```python
from build123d import *

# Parameters (mm, degrees)
SKETCH1_R           = 7.875
BOSS_EXTRUDE1_DEPTH = 1
SKETCH2_R           = 0.85
CUT_EXTRUDE1_DEPTH  = 12.181737343
SKETCH3_R           = 0.65
CUT_EXTRUDE2_DEPTH  = 11


with BuildPart() as part:
    # Sketch1 → Boss-Extrude1 (new body)
    with BuildSketch(Plane(origin=(0, 0, 0), x_dir=(1, 0, 0), z_dir=(0, 1, 0))):
        with Locations(Location((0, 0, 0), (0, 0, 270))):
            Circle(SKETCH1_R)
    extrude(amount=BOSS_EXTRUDE1_DEPTH)

    # Sketch2 → Cut-Extrude1 (cut, through all)
    with BuildSketch(Plane(origin=(0, 1, 0), x_dir=(1, 0, 0), z_dir=(0, 1, 0))):
        with Locations(Location((0, 6.125, 0), (0, 0, 270))):
            Circle(SKETCH2_R)
        with Locations(Location((0, -6.125, 0), (0, 0, 90))):
            Circle(SKETCH2_R)
    extrude(amount=-CUT_EXTRUDE1_DEPTH, mode=Mode.SUBTRACT)

    # Sketch3 → Cut-Extrude2 (cut)
    with BuildSketch(Plane(origin=(0, 1, 0), x_dir=(1, 0, 0), z_dir=(0, 1, 0))):
        with Locations(Location((0.503115295, 1.65, 0), (0, 0, 270))):
            Circle(SKETCH3_R)
        with Locations(Location((0.503115295, -1.65, 0), (0, 0, 270))):
            Circle(SKETCH3_R)
    extrude(amount=-CUT_EXTRUDE2_DEPTH, mode=Mode.SUBTRACT)


solid = part.part
```
Part model, mm, in its own coordinate system. Round coordinates to 2 decimals unless told otherwise and drop trailing zeros. Order: outer loops, then holes, each group sorted by start corner. A loop starts at its lowest first (then second) coordinate and runs counter-clockwise, first axis right, second up. Notation, with made-up numbers: M 42.5,-11 L 91.5,-11 A14 cw 91.5,-6 Z; hole C 5,78 d7. An arc over 180 degrees is marked long. Answer in a Markdown table with one row per item. Add a question column.
Q1. Cut at B-B on y = 0.75. Give the cut face in (x, z) (3 decimals).
Q2. Cut at A-A on z = -5.5. Give the cut face in (x, y), and give its area (3 significant figures).
Q3. Cut at C-C on z = 6.5. Give the cut face in (x, y).
Q4. Wall check: L1, parallel to X at y = 0.35, z = -1.65; L2, parallel to X at y = 0.2, z = 6.25; L3, parallel to Z at x = -5.25, y = 0.45. Give the ranges that are in metal, low to high. Write a range as from..to.
Q5. Cut at D-D on x = 3.5. Give the cut face in (y, z).
Q6. Mould opens along X. For faces 1 (the face through (0, 0, 0)), 2 (the face through (-0.255, 0.507, 5.314)), 3 (the face through (7.808, 0.493, -1.025)) say: +X half, -X half, draft (parallel to the pull), parting line (faces both ways), or undercut.
Established:
| question | item | result |
|---|---|---|
| 1 | outline | C 0,0 d15.75; hole C 0,-6.125 d1.7; hole C 0,6.125 d1.7; hole C 0.503,-1.65 d1.3; hole C 0.503,1.65 d1.3 |
| 2 | outline | M -5.64,0 L -0.58,0 L -0.58,1 L -5.64,1 Z; M 0.58,0 L 5.64,0 L 5.64,1 L 0.58,1 Z |
| 2 | area | 10.1 mm2 |
| 3 | outline | M -4.45,0 L -0.76,0 L -0.76,1 L -4.45,1 Z; M 0.76,0 L 4.45,0 L 4.45,1 L 0.76,1 Z |
| 4 | L1 | x = -7.7..-0.15, 1.15..7.7 |
| 4 | L2 | x = -4.79..-0.84, 0.84..4.79 |
| 4 | L3 | z = -5.87..5.87 |
| 5 | outline | M 0,-7.05 L 1,-7.05 L 1,7.05 L 0,7.05 Z |
| 6 | face 1 | draft |
| 6 | face 2 | undercut |
| 6 | face 3 | parting line |
